Read the model definition and answer for the solid it produces. Units are mm, in the model's axes. Face numbers are marked on the shaded views. A direction names the side the tool comes from. Round coordinates to 2 decimals unless told otherwise and drop trailing zeros. Order: outer loops, then holes, each group sorted by start corner. A loop starts at its lowest first (then second) coordinate and runs counter-clockwise, first axis right, second up.
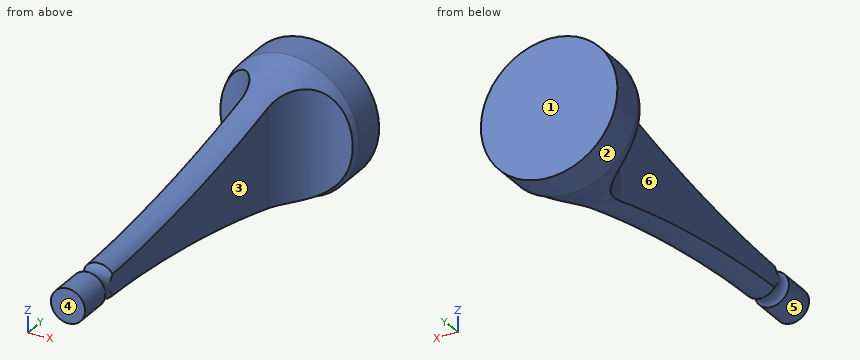
from build123d import *

# Parameters (mm, degrees)
F3_DEPTH      = 10.001
F3_DEPTH_BACK = 82


# Not quite as in the source:
# - an extrude ends at something that could not be found from the text; its depth is read off the source's solid


with BuildPart() as f1:
    # F0 (on Right) → F1 (revolve)
    with BuildSketch(Plane.YZ):
        with BuildLine():
            Line((-60, 0), (0, 0))
            Line((0, 0), (0, 10))
            Line((0, 10), (-5, 10))
            ThreePointArc((-5, 10), (-28.4012730043, 4.5885703785), (-52.3309178064, 2.5209029927))
            ThreePointArc((-52.3309178064, 2.5209029927), (-53.6614617682, 2.00006133), (-55, 2.5))
            Line((-55, 2.5), (-60, 2.5))
            Line((-60, 2.5), (-60, 0))
        make_face()
    revolve(axis=Axis((0, -19.4839663044, 0), (0, -1, 0)))

    # F2 (on Top) → F3 (cut, two sides)
    with BuildSketch(Plane.XY) as f3_sk:
        with BuildLine():
            Line((2, -14), (2, -53.5))
            Line((2, -53.5), (10, -53.5))
            Line((10, -53.5), (10, -6))
            ThreePointArc((10, -6), (4.3431457505, -8.3431457505), (2, -14))
        make_face()
        with BuildLine():
            Line((-10, -53.5), (-2, -53.5))
            Line((-2, -53.5), (-2, -14))
            ThreePointArc((-2, -14), (-4.3431457505, -8.3431457505), (-10, -6))
            Line((-10, -6), (-10, -53.5))
        make_face()
    extrude(amount=-F3_DEPTH, mode=Mode.SUBTRACT)
    extrude(f3_sk.sketch, amount=F3_DEPTH_BACK, mode=Mode.SUBTRACT)


solid = f1.part
Q1. For the marked faces 5 and 6, determine the directions among +Z, -Z, +X, -X, +Y, -Y from which every point of the face is accessible in a straight line to the end or side of a thin tool.
Outcome:
face 5: -Y
face 6: +Z, -Z, -X
Q2. Flat-ended cylindrical pins translate along their axes: pin 1 (6 mm diameter, centred on y = -44.5, z = -7, fed in from -X); pin 2 (12 mm diameter, centred on y = -51, z = -3, fed in from +X); pin 3 (1.5 mm diameter, centred on x = -5.5, z = 5, fed in from +Y); pin 4 (8 mm diameter, centred on y = -14, z = 2.5, fed in from -X). Find the tip coordinate at first contact, or state that the pin passes through.
Outcome:
pin 1: passes through
pin 2: stops at x = 2.5
pin 3: stops at y = 0
pin 4: stops at x = -3.07
Q3. A cutting plane is placed at A-A, the plane x = 0. Give the vertices of the cut face in (y, z), plus the area to 3 significant figures.
Outcome:
outline: (-60, -2.5) - (-55, -2.5) arc R2 cw to (-52.33, -2.52) arc R170.42 cw to (-5, -10) - (0, -10) - (0, 10) - (-5, 10) arc R170.42 cw to (-52.33, 2.52) arc R2 cw to (-55, 2.5) - (-60, 2.5) - close
area: 621 mm2
Q4. For a pull along Y with two mould halves and no side action, classify the marked faces 1, 2, 3 and 4 as released by +Y, released by -Y, zero draft, split by the parting line, or undercut.
Outcome:
face 1: released by +Y
face 2: zero draft
face 3: undercut
face 4: released by -Y
Q5. A cutting plane is placed at B-B, the plane y = -50. Give the vertices of the cut face in (x, z), plus the area to 3 significant figures.
Outcome:
outline: (-2, -1.62) arc R2.57 ccw to (2, -1.62) - (2, 1.62) arc R2.57 ccw to (-2, 1.62) - close
area: 18.3 mm2
Q6. Straight lines are drawn through the part: probe 1 along Z at (x, y) = (0.5, -3.5); probe 2 along X at (y, z) = (-15, -4.5); probe 3 along Y at (x, z) = (5, -7.5) (3 decimals). For each, find the intervals that lie inside material, in ascending order.
Outcome:
probe 1: z = -9.99 to 9.99
probe 2: x = -2 to 2
probe 3: y = -7.755 to 0
